Input: dimensioned drawing with shaded views. Units: mm. Origin: part minimum x, y, z. Round coordinates to 2 decimals unless told otherwise and drop trailing zeros. Loops run counter-clockwise (first coordinate to the right, second up) from the corner with the lowest first, then second, coordinate; pieces in that order, holes last. Notation, with made-up numbers: M 85.25,-2 L 115.25,-2 A32 ccw 115.25,28 Z; hole C 65.5,-9 d2. An arc over 180 degrees is marked long. Answer as a JSON object with one key per item and string values.
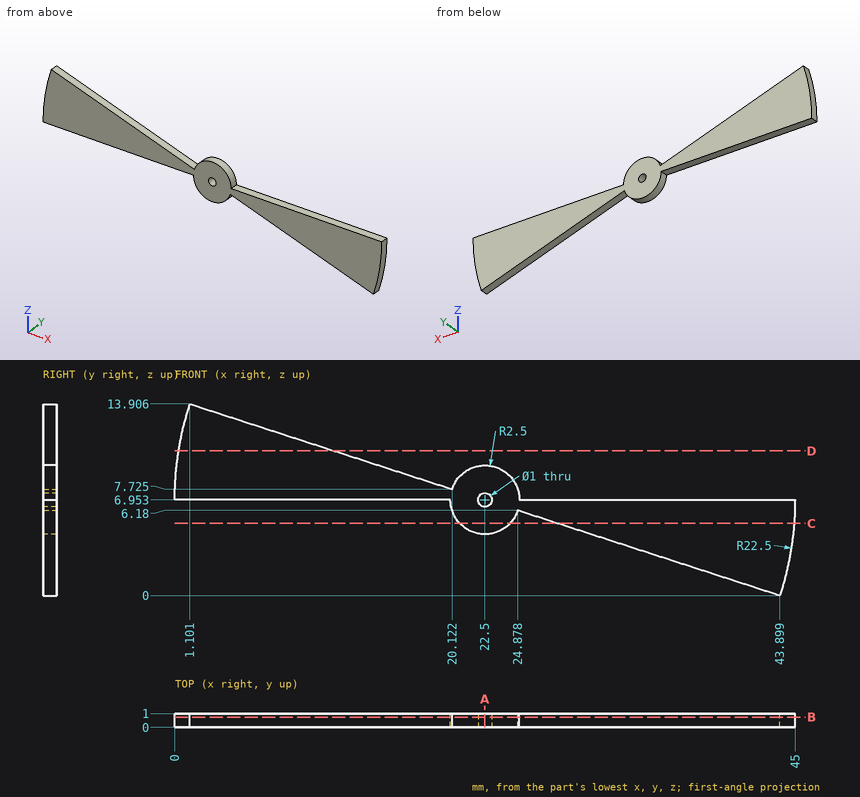
Item 1: Line query: probe 1 along Z at (x, y) = (40, 0.55); probe 2 along Z at (x, y) = (38.5, 0.6) (1 decimal); probe 3 along X at (y, z) = (0.6, 6.25). Output: solid intervals per line, ascending. Write a range as from..to.
Answer sheet:
{"probe 1": "z = 1.27..6.95", "probe 2": "z = 1.8..7", "probe 3": "x = 20.1..44.99"}
Item 2: Section B-B on y = 0.75. Return the cut outline in (x, z) (1 decimal).
Answer sheet:
{"outline": "M 0,7 L 20,7 A2.5 ccw 24.9,6.2 L 43.9,0 A22.5 ccw 45,7 L 25,7 A2.5 ccw 20.1,7.7 L 1.1,13.9 A22.5 ccw Z; hole C 22.5,7 d1"}
Item 3: Section C-C on z = 5.25. Return the cut outline in (x, y) (1 decimal).
Answer sheet:
{"outline": "M 20.7,0 L 24.3,0 L 24.3,1 L 20.7,1 Z; M 27.7,0 L 44.9,0 L 44.9,1 L 27.7,1 Z"}
Item 4: Section A-A on x = 22.5. Return the cut outline in (y, z).
Answer sheet:
{"outline": "M 0,4.45 L 1,4.45 L 1,6.45 L 0,6.45 Z; M 0,7.45 L 1,7.45 L 1,9.45 L 0,9.45 Z"}
Item 5: Section D-D on z = 10.5. Return the cut outline in (x, y).
Answer sheet:
{"outline": "M 0.28,0 L 11.58,0 L 11.58,1 L 0.28,1 Z"}
